For this review, take the finished solid that the model builds, in its own axes (mm). A direction names the side the tool comes from. Round coordinates to 2 decimals unless told otherwise and drop trailing zeros. Loops run counter-clockwise (first coordinate to the right, second up) from the corner with the lowest first, then second, coordinate; pieces in that order, holes last. Notation, with made-up numbers: M 31.5,-4 L 57.5,-4 A10 cw 57.5,1 Z; hole C -33,-1 d6. An arc over 180 degrees is marked long. One line per question, with ' | ' between items. Start each with the question number.
1) We need section C-C (x = -0.5). Give the boundary of the cut face in (y, z).
2) Mouldability with a two-part tool opening along Z and no side actions: class faces 4 (the face through (3.57, 3.763, 5.676)), 5 (the face through (3.5, -6.07, 5.03)), 6 (the face through (0, -3, 2.6)) as pulls with the +Z half, pulls with the -Z half, needs draft (parallel to the pull), parting line crosses it, or undercut.
3) For faces 1 (the face through (0, 0, 5)), 2 (the face through (4, 0, 9)), 3 (the face through (-4, 0, 1)), list the 3-axis set-ups (+Z, -Z, +X, -X, +Y, -Y) from which the entire face can be reached by the end or side of a thin tool; tool diameter is ignored.
4) We need section A-A (z = 5.5). State how many separate pieces and enclosed holes the cut face has, and give its area (3 significant figures).
5) For probe 1 along Y at (x, z) = (0, 4.35); probe 2 along X at (y, z) = (6, 5); probe 3 along Y at (x, z) = (3.75, 9), list the stretches that pass through material, from the lowest coordinate up. Write a range as from..to.
6) We need section D-D (y = 4.25). Give the boundary of the cut face in (x, z), and give its area (3 significant figures).
7) We need section B-B (y = 0.5). Give the boundary of the cut face in (x, z), and give its area (3 significant figures).
8) For pin 1 Ø3.5 at (x, z) = (-0.5, 6) entering from +Y; pin 2 Ø3 at (x, y) = (0, -4.5) entering from +Z; pin 3 Ø2 at (x, z) = (4, 1.5) entering from -Y, all flat-tipped, find the tip position at first contact; note any pin that passes through.
```python
from build123d import *

# Parameters (mm, degrees)
SKETCH1_R           = 1
BOSS_EXTRUDE1_DEPTH = 10
SKETCH2_R           = 1
SKETCH2_W           = 2.6
SKETCH2_H           = 7.5
CUT_EXTRUDE1_DEPTH  = 10
FILLET1_R           = 5


with BuildPart() as part:
    # Sketch1 → Boss-Extrude1 (new body)
    with BuildSketch(Plane.XY):
        Polygon((-5, -7.5), (5, -7.5), (5, 7.5), (2.1, 7.5), (2.1, 0), (-2.1, 0), (-2.1, 7.5), (-5, 7.5), align=None)
        with Locations((0, -4.5)):
            Circle(SKETCH1_R, mode=Mode.SUBTRACT)
    extrude(amount=BOSS_EXTRUDE1_DEPTH)

    # Sketch2 → Cut-Extrude1 (cut)
    with BuildSketch(Plane(origin=(5, 0, 0), x_dir=(0, 0, -1), z_dir=(1, 0, 0))):
        with Locations(Location((-5, 4.5, 0), (0, 0, 90))):
            Circle(SKETCH2_R)
        with Locations((-8.7, -3.75)):
            Rectangle(SKETCH2_W, SKETCH2_H)
        with Locations((-1.3, -3.75)):
            Rectangle(SKETCH2_W, SKETCH2_H)
    extrude(amount=-CUT_EXTRUDE1_DEPTH, mode=Mode.SUBTRACT)

    # Fillet1
    fillet1_edges = [part.edges().sort_by_distance(p)[0] for p in [
        (-5, -7.5, 5),
        (5, -7.5, 5),
        (-3.55, 7.5, 0),
        (3.55, 7.5, 0),
        (3.55, 7.5, 10),
        (-3.55, 7.5, 10),
    ]]
    fillet(fillet1_edges, radius=FILLET1_R - 0.0001)  # a hair under: the kernel refuses the full size


solid = part.part
```
Answers below:
1) outline: M -7.47,2.6 L -5.37,2.6 L -5.37,7.4 L -7.47,7.4 Z; M -3.63,2.6 L 0,2.6 L 0,7.4 L -3.63,7.4 Z
2) face 4: undercut | face 5: needs draft | face 6: pulls with the -Z half
3) face 1: +Z, -Z, +Y | face 2: +Z, +X, -X, -Y | face 3: -Z, +X, -X, -Y
4) separate pieces: 3 | enclosed holes: 1 | area: 94.4 mm^2
5) probe 1: -7.5..-5.5, -3.5..0 | probe 2: -5..-2.1, 2.1..5 | probe 3: 0..5.5
6) outline: M -5,0.32 L -2.1,0.32 L -2.1,4.03 L -5,4.03 Z; M -5,5.97 L -2.1,5.97 L -2.1,9.68 L -5,9.68 Z; M 2.1,0.32 L 5,0.32 L 5,4.03 L 2.1,4.03 Z; M 2.1,5.97 L 5,5.97 L 5,9.68 L 2.1,9.68 Z | area: 43.1 mm^2
7) outline: M -5,0 L -2.1,0 L -2.1,10 L -5,10 Z; M 2.1,0 L 5,0 L 5,10 L 2.1,10 Z | area: 58.0 mm^2
8) pin 1: y = 7.49 | pin 2: z = 7.4 | pin 3: y = 0
